from build123d import *

# Parameters (mm, degrees)
F0_R     = 12.7
F1_DEPTH = 50.8
F2_D     = 8.255


with BuildPart() as f1:
    # F0 (on Front) → F1 (new body)
    with BuildSketch(Plane.XZ):
        with BuildLine():
            ThreePointArc((73.603548, 19.722011), (-75.548098, -9.946096), (76.2, 0))
            ThreePointArc((76.2, 0), (75.548098, 9.946096), (73.603548, 19.722011))
        make_face()
        with BuildLine():
            Line((24.534516, -6.574004), (61.33629, -16.435009))
            ThreePointArc((61.33629, -16.435009), (31.75, -54.992613), (-16.435009, -61.33629))
            Line((-16.435009, -61.33629), (-6.574004, -24.534516))
            ThreePointArc((-6.574004, -24.534516), (12.7, -21.997045), (24.534516, -6.574004))
        make_face(mode=Mode.SUBTRACT)
        with BuildLine():
            ThreePointArc((-44.901281, -44.901281), (-63.5, 0), (-44.901281, 44.901281))
            Line((-44.901281, 44.901281), (-17.960512, 17.960512))
            ThreePointArc((-17.960512, 17.960512), (-25.4, 0), (-17.960512, -17.960512))
            Line((-17.960512, -17.960512), (-44.901281, -44.901281))
        make_face(mode=Mode.SUBTRACT)
        Circle(F0_R, mode=Mode.SUBTRACT)
        with BuildLine():
            ThreePointArc((-16.435009, 61.33629), (31.75, 54.992613), (61.33629, 16.435009))
            Line((61.33629, 16.435009), (24.534516, 6.574004))
            ThreePointArc((24.534516, 6.574004), (12.7, 21.997045), (-6.574004, 24.534516))
            Line((-6.574004, 24.534516), (-16.435009, 61.33629))
        make_face(mode=Mode.SUBTRACT)
    extrude(amount=F1_DEPTH)

    # F2 (through all)
    with Locations(Plane(origin=(0, 0, 0), x_dir=(1, 0, 0), z_dir=(0, 1, 0))):
        with Locations((47.625, 0), (-23.8125, -41.24446), (-23.8125, 41.24446)):
            Hole(F2_D / 2)


solid = f1.part
Could you check a few things on this model? Use its own coordinates, in mm. A direction names the side the tool comes from. Coordinates: 2 decimals unless noted, no trailing zeros. Write each loop counter-clockwise with the first axis right and the second up, starting at its lowest first coordinate (ties: lowest second). Pieces come first, ordered by that corner, then holes. Notation, with made-up numbers: (-24, 75) - (35, 75) arc R13 ccw to (35, 100) - close; hole circle Ø6 at (-8.75, 18.5). An arc over 180 degrees is marked (long way). Put each result on its own line as item: value. Start each with the question number.
Q1. I want a section at B-B on z = 31. Write out the boundary of the cut face in (x, y), plus the area to 3 significant figures.
Q2. Which directions (+Z, -Z, +X, -X, +Y, -Y) give clear straight access to the entire face, cutting with the end or side of a thin tool? Please do faces 5 (the flat face through (-1, -50.8, -16)), 6 (the cylindrical face through (12.941, -25.044, 21.856)).
Q3. I want a section at D-D on x = -47.5. Write out the boundary of the cut face in (y, z).
Q4. I want a section at C-C on x = 0. Write out the boundary of the cut face in (y, z), plus the area to 3 significant figures.
Q5. Please list where these lines run through material, in increasing order: L1, parallel to X at y = -15.5, z = -38.5; L2, parallel to X at y = -14, z = -18; L3, parallel to Z at x = 42, y = -20.
Q6. I want a section at A-A on x = 33.5. Write out the boundary of the cut face in (y, z).
Q7. Thinking about a two-plate mould opening in X: for faces 1 (the cylindrical face through (32.35, -25.04, -54.64)), 2 (the cylindrical face through (75.566, -25.044, 9.808)), 3 (the flat face through (-1, 0, -16)), 4 (the cylindrical face through (-75.9, -25.04, -6.75)), which applies, pulls with the +X half, pulls with the -X half, needs draft (parallel to the pull), parting line crosses it, or undercut?
Q8. I'm going to push flat-ended pins straight in: P1, Ø2, axis at y = -7, z = -56.5, coming from the -X side; P2, Ø10, axis at y = -30, z = 56, coming from the +X side; P3, Ø1, axis at x = -20, y = -9.5, coming from the +Z side. Where does each tip first touch, or does it pass through?
Checks:
1. outline: (-69.61, -50.8) - (-55.42, -50.8) - (-55.42, 0) - (-69.61, 0) - close; (-31, -50.8) - (-8.31, -50.8) - (-8.31, 0) - (-31, 0) - close; (55.42, -50.8) - (69.61, -50.8) - (69.61, 0) - (55.42, 0) - close
1. area: 2,590 mm²
2. face 5: +Z, -Z, +X, -X, -Y
2. face 6: +Y, -Y
3. outline: (-50.8, -59.58) - (0, -59.58) - (0, -42.14) - (-50.8, -42.14) - close; (-50.8, 42.14) - (0, 42.14) - (0, 59.58) - (-50.8, 59.58) - close
4. outline: (-50.8, -76.2) - (0, -76.2) - (0, -63.5) - (-50.8, -63.5) - close; (-50.8, -25.4) - (0, -25.4) - (0, -12.7) - (-50.8, -12.7) - close; (-50.8, 12.7) - (0, 12.7) - (0, 25.4) - (-50.8, 25.4) - close; (-50.8, 63.5) - (0, 63.5) - (0, 76.2) - (-50.8, 76.2) - close
4. area: 2,580 mm²
5. L1: -65.76 to -50.5, -38.5 to -26.9, -20.73 to -10.32, 50.5 to 65.76
5. L2: -74.04 to -60.9, -18 to 17.92, 60.9 to 74.04
5. L3: -63.58 to -47.63, -11.25 to 11.25, 47.63 to 63.58
6. outline: (-50.8, -68.44) - (0, -68.44) - (0, -53.94) - (-50.8, -53.94) - close; (-50.8, -8.98) - (0, -8.98) - (0, 8.98) - (-50.8, 8.98) - close; (-50.8, 53.94) - (0, 53.94) - (0, 68.44) - (-50.8, 68.44) - close
7. face 1: undercut
7. face 2: pulls with the +X half
7. face 3: needs draft
7. face 4: parting line crosses it
8. P1: x = -52.21
8. P2: x = 56.62
8. P3: z = 73.66
